Here's how the part is built. I have some questions about the finished solid (model axes, mm). A direction names the side the tool comes from. Round coordinates to 2 decimals unless told otherwise and drop trailing zeros. Write each loop counter-clockwise with the first axis right and the second up, starting at its lowest first coordinate (ties: lowest second). Pieces come first, ordered by that corner, then holes. Notation, with made-up numbers: (-29, -18) - (18, -18) arc R15 ccw to (18, -12) - close; hole circle Ø5 at (-29.5, -4). An arc over 180 degrees is marked (long way). One line per item, written item: value. Start each with the question number.
Item 1: For P1, Ø12.5, axis at x = 33.5, y = 24, coming from the +Z side; P2, Ø2, axis at y = 43.5, z = 41, coming from the +X side; P3, Ø7, axis at y = 19.5, z = 4, coming from the +X side, each with a flat end and sliding along its axis, tell me the tip position at first contact or that it passes through.
Item 2: Imagine slicing it at D-D, the plane x = 22. Please give me the cut outline in (y, z), then the cut area to 3 significant figures.
Item 3: Imagine slicing it at B-B, the plane y = 36.65. Please give me the cut outline in (x, z).
Item 4: If I drill on line 1 (Y direction, x = 10.35, z = 6.5); line 2 (Y direction, x = 10, z = 2); line 3 (X direction, y = 43.2, z = 19), over which ranges is the centre line in solid material (lowest first)?
Item 5: Imagine slicing it at C-C, the plane x = 10. Please give me the cut outline in (y, z).
Item 6: Thinking about a two-plate mould opening in X: for faces 1 (the face through (0.9, 22.31, 0.86)), 2 (the face through (26.14, 46.1, 38.65)), 3 (the face through (17.715, 27.107, 4.563)), which applies, released by +X, released by -X, zero draft, split by the parting line, or undercut?
Item 7: Imagine slicing it at A-A, the plane z = 6.5. Please give me the cut outline in (x, y).
Item 8: For faces 4 (the face through (40, 43, 19)), 5 (the face through (27, 43, 40)), 6 (the face through (11, 7, 5)), 7 (the face through (47, 38, 8)), 8 (the face through (10, 21, 5)), which set-ups out of +Z, -Z, +X, -X, +Y, -Y let a thin tool reach every point of the face, with its end or its side?
```python
from build123d import *

# Parameters (mm, degrees)
BOSS_EXTRUDE1_DEPTH = 9
SKETCH3_R           = 1.5
CUT_EXTRUDE1_DEPTH  = 10
SKETCH4_W           = 5
SKETCH4_H           = 47
BOSS_EXTRUDE2_DEPTH = 38
CUT_EXTRUDE2_DEPTH  = 38
SKETCH6_W           = 42
SKETCH6_H           = 5
BOSS_EXTRUDE3_DEPTH = 38
SKETCH7_R           = 4
CUT_EXTRUDE3_DEPTH  = 5
CUT_EXTRUDE4_DEPTH  = 10
FILLET1_R           = 3
SKETCH9_R           = 1.5
CUT_EXTRUDE5_DEPTH  = 10
SKETCH10_R          = 3
CUT_EXTRUDE6_DEPTH  = 2


with BuildPart() as part:
    # Sketch2 → Boss-Extrude1 (new body)
    with BuildSketch(Plane.XY):
        with BuildLine():
            Line((0, 0), (0, 47))
            Line((0, 47), (47, 47))
            Line((47, 47), (47, 25.75))
            Line((47, 25.75), (31.68, 25.75))
            ThreePointArc((31.68, 25.75), (24.5283031, 28.175540714), (17, 27.58))
            Line((17, 27.58), (17, 0))
            Line((17, 0), (0, 0))
        make_face()
    extrude(amount=BOSS_EXTRUDE1_DEPTH)

    # Sketch3 → Cut-Extrude1 (cut)
    with BuildSketch(Plane.XY.offset(9)):
        with Locations((10.35, 5.65)):
            Circle(SKETCH3_R)
        with Locations((10.35, 36.65)):
            Circle(SKETCH3_R)
        with Locations((41.35, 36.65)):
            Circle(SKETCH3_R)
    extrude(amount=-CUT_EXTRUDE1_DEPTH, mode=Mode.SUBTRACT)

    # Sketch4 → Boss-Extrude2 (add)
    with BuildSketch(Plane.XY.offset(9)):
        with Locations((2.5, 23.5)):
            Rectangle(SKETCH4_W, SKETCH4_H)
    extrude(amount=BOSS_EXTRUDE2_DEPTH)

    # Sketch5 → Cut-Extrude2 (cut)
    with BuildSketch(Plane.ZY):
        Polygon((47, 32), (32, 32), (9, 0), (47, 0), align=None)
    extrude(amount=-CUT_EXTRUDE2_DEPTH, mode=Mode.SUBTRACT)

    # Sketch6 → Boss-Extrude3 (add)
    with BuildSketch(Plane.XY.offset(9)):
        with Locations((26, 44.5)):
            Rectangle(SKETCH6_W, SKETCH6_H)
    extrude(amount=BOSS_EXTRUDE3_DEPTH)

    # Sketch7 → Cut-Extrude3 (cut)
    with BuildSketch(Plane(origin=(0, 0, 0), x_dir=(-1, 0, 0), z_dir=(0, 0, -1))):
        with Locations((-10, 20.85)):
            Circle(SKETCH7_R)
    extrude(amount=-CUT_EXTRUDE3_DEPTH, mode=Mode.SUBTRACT)

    # Sketch8 → Cut-Extrude4 (cut)
    with BuildSketch(Plane(origin=(0, 42, 0), x_dir=(-1, 0, 0), z_dir=(0, -1, 0))):
        Polygon((-27, -32), (-47, -23), (-47, -47), (-27, -47), align=None)
    extrude(amount=-CUT_EXTRUDE4_DEPTH, mode=Mode.SUBTRACT)

    # Fillet1
    fillet1_edges = [part.edges().sort_by_distance(p)[0] for p in [
        (0, 47, 23.5),
        (47, 25.75, 4.5),
        (17, 27.58, 4.5),
        (17, 0, 4.5),
        (0, 0, 4.5),
        (0, 32, 39.5),
        (0, 16, 20.5),
        (0, 23.5, 0),
        (23.5, 47, 0),
        (47, 36.375, 0),
        (13.5, 47, 47),
        (47, 47, 11.5),
        (27, 47, 39.5),
        (37, 47, 27.5),
    ]]
    fillet(fillet1_edges, radius=FILLET1_R)

    # Sketch9 → Cut-Extrude5 (cut)
    with BuildSketch(Plane(origin=(0, 42, 0), x_dir=(-1, 0, 0), z_dir=(0, -1, 0))):
        with Locations((-37, -19)):
            Circle(SKETCH9_R)
    extrude(amount=-CUT_EXTRUDE5_DEPTH, mode=Mode.SUBTRACT)

    # Sketch10 → Cut-Extrude6 (cut)
    with BuildSketch(Plane(origin=(0, 42, 0), x_dir=(-1, 0, 0), z_dir=(0, -1, 0))):
        with Locations((-37, -19)):
            Circle(SKETCH10_R)
    extrude(amount=-CUT_EXTRUDE6_DEPTH, mode=Mode.SUBTRACT)


solid = part.part
```
Values follow:
1. P1: stops at z = 9
1. P2: stops at x = 27
1. P3: stops at x = 17
2. outline: (28.32, 0) - (44, 0) arc R3 ccw to (47, 3) - (47, 44) arc R3 ccw to (44, 47) - (42, 47) - (42, 9) - (28.32, 9) - close
2. area: 354 mm^2
3. outline: (0, 3) arc R3 ccw to (3, 0) - (8.85, 0) - (8.85, 9) - (5, 9) - (5, 47) - (0, 47) - close; (11.85, 0) - (39.85, 0) - (39.85, 9) - (11.85, 9) - close; (42.85, 0) - (44, 0) arc R3 ccw to (47, 3) - (47, 9) - (42.85, 9) - close
4. line 1: y = 0 to 4.15, 7.15 to 35.15, 38.15 to 47
4. line 2: y = 0 to 4.19, 7.11 to 16.85, 24.85 to 35.19, 38.11 to 46.83
4. line 3: x = 0 to 34, 40 to 47
5. outline: (0, 0) - (4.19, 0) - (4.19, 9) - (0, 9) - close; (7.11, 0) - (16.85, 0) - (16.85, 5) - (24.85, 5) - (24.85, 0) - (35.19, 0) - (35.19, 9) - (7.11, 9) - close; (38.11, 0) - (44, 0) arc R3 ccw to (47, 3) - (47, 44) arc R3 ccw to (44, 47) - (42, 47) - (42, 9) - (38.11, 9) - close
6. face 1: released by -X
6. face 2: released by +X
6. face 3: undercut
7. outline: (0, 3) arc R3 ccw to (3, 0) - (14, 0) arc R3 ccw to (17, 3) - (17, 25.16) arc R3 cw to (19.58, 28.13) arc R18.73 cw to (31.68, 25.75) - (44, 25.75) arc R3 ccw to (47, 28.75) - (47, 44) arc R3 ccw to (44, 47) - (3, 47) arc R3 ccw to (0, 44) - close; hole circle Ø3 at (10.35, 5.65); hole circle Ø3 at (10.35, 36.65); hole circle Ø3 at (41.35, 36.65)
8. face 4: -Y
8. face 5: +Z, +X, +Y, -Y
8. face 6: +Z, -Z
8. face 7: +Z, -Z, +X, +Y, -Y
8. face 8: -Z
